For this review, take the finished solid that the model builds, in its own axes (mm). A direction names the side the tool comes from. Round coordinates to 2 decimals unless told otherwise and drop trailing zeros. Order: outer loops, then holes, each group sorted by start corner. A loop starts at its lowest first (then second) coordinate and runs counter-clockwise, first axis right, second up. Notation, with made-up numbers: (48, -18.5) -> (89, -18.5) arc R25 cw to (89, 6.5) -> close; hole circle Ø8 at (1.5, -22.75). An arc over 180 degrees is marked (long way). Use a Markdown table: item, result. Add a question column.
1) Consider section A-A (x = 5). State the section outline as (y, z) points, plus the area to 3 significant figures.
2) Consider section B-B (y = 29). State the section outline as (x, z) points, plus the area to 3 significant figures.
3) Wall thickness on line 1 along X through (y, z) = (36.5, 5); line 2 along Z through (x, y) = (-26.55, 10.1); line 3 along Z through (x, y) = (26.6, 17.1): over which ranges is each line inside the solid? List them lowest first. Write a range as [from, to].
4) Clearance check with flat-ended pins moving along their axes: P1, Ø4, axis at y = 15.05, z = 4.95, coming from the -X side; P2, Ø2.5, axis at x = 15, z = -5, coming from the -Y side; P3, Ø5, axis at x = 5, z = -5, coming from the -Y side. State where each tip first meets the part, or that it passes through.
5) Consider section C-C (z = -2.25). State the section outline as (x, y) points.
6) Machinability: for faces 4 (the face through (26.789, 4.486, -0.575)), 5 (the face through (-25.8, 22, 0)), which of the approach directions +Z, -Z, +X, -X, +Y, -Y give a long, thin tool a straight path to every point of the face, cutting with its end or side? Answer none if there is none.
7) Draft analysis for pull direction X (two halves, no side actions). For faces 1 (the face through (0.9, 35.94, 2.86)), 2 (the face through (16.586, 35.939, -5.208)), 3 (the face through (26.79, 15.6, 0.07)), state which applies: pulls with the +X half, pulls with the -X half, needs draft (parallel to the pull), parting line crosses it, or undercut.
8) Consider section D-D (y = 3.1). State the section outline as (x, z) points.
```python
from build123d import *

# Parameters (mm, degrees)
BOSS_EXTRU_1_DEPTH      = 10.1
ENL_V_MAT_EXTRU_2_DEPTH = 68.408233918
ESQUISSE3_R             = 3
ESQUISSE3_R_2           = 1.6
ENL_V_MAT_EXTRU_1_DEPTH = 48.261850366
ESQUISSE5_R             = 4
ESQUISSE5_R_2           = 1.5
ENL_V_MAT_EXTRU_3_DEPTH = 68.408233918


with BuildPart() as part:
    # Esquisse1 → Boss.-Extru.1 (new, symmetric)
    with BuildSketch(Plane.XY):
        Polygon((-27.75, 36.9), (27.75, 36.9), (27.75, 0), (25.8, 0), (25.8, 34.95), (-25.8, 34.95), (-25.8, 0), (-27.75, 0), align=None)
    extrude(amount=BOSS_EXTRU_1_DEPTH, both=True)

    # Esquisse4 → Enlèv. mat.-Extru.2 (cut, through all)
    with BuildSketch(Plane(origin=(27.75, 0, 0), x_dir=(0, 0, -1), z_dir=(1, 0, 0))):
        with BuildLine():
            ThreePointArc((0, 0), (-7.14177849, 2.95822151), (-10.1, 10.1))
            Line((-10.1, 10.1), (-10.1, 0))
            Line((-10.1, 0), (0, 0))
        make_face()
        with BuildLine():
            ThreePointArc((10.1, 10.1), (7.14177849, 2.95822151), (0, 0))
            Line((0, 0), (10.1, 0))
            Line((10.1, 0), (10.1, 10.1))
        make_face()
    extrude(amount=-ENL_V_MAT_EXTRU_2_DEPTH, mode=Mode.SUBTRACT)

    # Esquisse3 → Enlèv. mat.-Extru.1 (cut, through all)
    with BuildSketch(Plane(origin=(0, 36.9, 0), x_dir=(1, 0, 0), z_dir=(0, 1, 0))):
        with Locations(Location((0, 0, 0), (0, 0, 270))):
            Circle(ESQUISSE3_R)
        with Locations(Location((-5, 5, 0), (0, 0, 270))):
            Circle(ESQUISSE3_R_2)
        with Locations(Location((-5, -5, 0), (0, 0, 270))):
            Circle(ESQUISSE3_R_2)
        with Locations(Location((5, -5, 0), (0, 0, 270))):
            Circle(ESQUISSE3_R_2)
        with Locations(Location((5, 5, 0), (0, 0, 270))):
            Circle(ESQUISSE3_R_2)
        with Locations(Location((-15, 5, 0), (0, 0, 270))):
            Circle(ESQUISSE3_R_2)
        with Locations(Location((-15, -5, 0), (0, 0, 270))):
            Circle(ESQUISSE3_R_2)
        with Locations(Location((15, -5, 0), (0, 0, 270))):
            Circle(ESQUISSE3_R_2)
        with Locations(Location((15, 5, 0), (0, 0, 270))):
            Circle(ESQUISSE3_R_2)
    extrude(amount=-ENL_V_MAT_EXTRU_1_DEPTH, mode=Mode.SUBTRACT)

    # Esquisse5 → Enlèv. mat.-Extru.3 (cut, through all)
    with BuildSketch(Plane(origin=(27.75, 0, 0), x_dir=(0, 0, -1), z_dir=(1, 0, 0))):
        with Locations(Location((0, 10.1, 0), (0, 0, 90))):
            Circle(ESQUISSE5_R)
        with Locations(Location((-7, 10.1, 0), (0, 0, 90))):
            Circle(ESQUISSE5_R_2)
        with Locations(Location((-4.949747468, 15.049747468, 0), (0, 0, 90))):
            Circle(ESQUISSE5_R_2)
        with Locations(Location((0, 17.1, 0), (0, 0, 90))):
            Circle(ESQUISSE5_R_2)
        with Locations(Location((0, 3.1, 0), (0, 0, 90))):
            Circle(ESQUISSE5_R_2)
        with Locations(Location((7, 10.1, 0), (0, 0, 270))):
            Circle(ESQUISSE5_R_2)
        with Locations(Location((4.949747468, 15.049747468, 0), (0, 0, 270))):
            Circle(ESQUISSE5_R_2)
    extrude(amount=-ENL_V_MAT_EXTRU_3_DEPTH, mode=Mode.SUBTRACT)


solid = part.part
```
Results list:
| question | item | result |
|---|---|---|
| 1 | outline | (34.95, -10.1) -> (36.9, -10.1) -> (36.9, -6.6) -> (34.95, -6.6) -> close; (34.95, -3.4) -> (36.9, -3.4) -> (36.9, 3.4) -> (34.95, 3.4) -> close; (34.95, 6.6) -> (36.9, 6.6) -> (36.9, 10.1) -> (34.95, 10.1) -> close |
| 1 | area | 26.9 mm2 |
| 2 | outline | (-27.75, -10.1) -> (-25.8, -10.1) -> (-25.8, 10.1) -> (-27.75, 10.1) -> close; (25.8, -10.1) -> (27.75, -10.1) -> (27.75, 10.1) -> (25.8, 10.1) -> close |
| 2 | area | 78.8 mm2 |
| 3 | line 1 | [-27.75, -16.6], [-13.4, -6.6], [-3.4, 3.4], [6.6, 13.4], [16.6, 27.75] |
| 3 | line 2 | [-10.1, -8.5], [-5.5, -4], [4, 5.5], [8.5, 10.1] |
| 3 | line 3 | [-10.1, -1.5], [1.5, 10.1] |
| 4 | P1 | x = -27.75 |
| 4 | P2 | through |
| 4 | P3 | y = 34.95 |
| 5 | outline | (-27.75, 0.25) -> (-25.8, 0.25) -> (-25.8, 6.79) -> (-27.75, 6.79) -> close; (-27.75, 13.41) -> (-25.8, 13.41) -> (-25.8, 34.95) -> (-1.98, 34.95) -> (-1.98, 36.9) -> (-27.75, 36.9) -> close; (1.98, 34.95) -> (25.8, 34.95) -> (25.8, 13.41) -> (27.75, 13.41) -> (27.75, 36.9) -> (1.98, 36.9) -> close; (25.8, 0.25) -> (27.75, 0.25) -> (27.75, 6.79) -> (25.8, 6.79) -> close |
| 6 | face 4 | +X, -X |
| 6 | face 5 | +Z, -Z, -Y |
| 7 | face 1 | undercut |
| 7 | face 2 | undercut |
| 7 | face 3 | needs draft |
| 8 | outline | (-27.75, -7.28) -> (-25.8, -7.28) -> (-25.8, -1.5) -> (-27.75, -1.5) -> close; (-27.75, 1.5) -> (-25.8, 1.5) -> (-25.8, 7.28) -> (-27.75, 7.28) -> close; (25.8, -7.28) -> (27.75, -7.28) -> (27.75, -1.5) -> (25.8, -1.5) -> close; (25.8, 1.5) -> (27.75, 1.5) -> (27.75, 7.28) -> (25.8, 7.28) -> close |
